```python
from build123d import *

# Parameters (mm, degrees)
ESBO_O1_R                  = 25
RESSALTO_EXTRUS_O1_DEPTH   = 22
CORTE_EXTRUS_O1_DEPTH      = 24
CORTE_EXTRUS_O1_DEPTH_BACK = 32
CORTE_EXTRUS_O2_DEPTH      = 32
PADR_OCIRCULAR1_COUNT      = 14


with BuildPart() as part:
    # Esboço1 → Ressalto-extrusão1 (new body)
    with BuildSketch(Plane.XY):
        Circle(ESBO_O1_R)
    extrude(amount=RESSALTO_EXTRUS_O1_DEPTH)

    # Esboço2 → Corte-extrusão1 (cut, two sides: drawn at the far end of the back side and taken through both)
    with BuildSketch(Plane.XY.offset(22).offset(-CORTE_EXTRUS_O1_DEPTH_BACK)):
        with BuildLine():
            Line((-2.5, -11), (2.5, -11))
            Line((2.5, -11), (2.5, -14.282856857))
            ThreePointArc((2.5, -14.282856857), (10.253048327, -10.253048327), (14.282856857, -2.5))
            Line((14.282856857, -2.5), (11, -2.5))
            Line((11, -2.5), (11, 2.5))
            Line((11, 2.5), (14.282856857, 2.5))
            ThreePointArc((14.282856857, 2.5), (10.253048327, 10.253048327), (2.5, 14.282856857))
            Line((2.5, 14.282856857), (2.5, 11))
            Line((2.5, 11), (-2.5, 11))
            Line((-2.5, 11), (-2.5, 14.282856857))
            ThreePointArc((-2.5, 14.282856857), (-10.253048327, 10.253048327), (-14.282856857, 2.5))
            Line((-14.282856857, 2.5), (-11, 2.5))
            Line((-11, 2.5), (-11, -2.5))
            Line((-11, -2.5), (-14.282856857, -2.5))
            ThreePointArc((-14.282856857, -2.5), (-10.253048327, -10.253048327), (-2.5, -14.282856857))
            Line((-2.5, -14.282856857), (-2.5, -11))
        make_face()
    extrude(amount=CORTE_EXTRUS_O1_DEPTH + CORTE_EXTRUS_O1_DEPTH_BACK, mode=Mode.SUBTRACT)

    # Esboço3 → Corte-extrusão2 (cut)
    with BuildSketch(Plane.XY.offset(22)):
        Polygon((-3.376446492, -24.770942838), (0.890947549, -26.390974492), (3.376446492, -24.770942838), (2.5, -21.5), (-2.5, -21.5), align=None)
    corte_extrus_o2 = extrude(amount=-CORTE_EXTRUS_O2_DEPTH, mode=Mode.SUBTRACT)

    # PadrãoCircular1: Corte-extrusão2 ×14 about axis
    padr_ocircular1_axis = Axis((0, 0, 0), (0, 0, 1))
    for i in range(1, PADR_OCIRCULAR1_COUNT):
        add(corte_extrus_o2.rotate(padr_ocircular1_axis, i * 360 / PADR_OCIRCULAR1_COUNT), mode=Mode.SUBTRACT)


solid = part.part
```
Source: CAD feature listing. Evaluate the final solid. Frame: model axes, mm. A direction names the side the tool comes from. Round coordinates to 2 decimals unless told otherwise and drop trailing zeros. Loops run counter-clockwise (first coordinate to the right, second up) from the corner with the lowest first, then second, coordinate; pieces in that order, holes last.
1. Ray query, L1, parallel to Y at x = 17, z = 14.75; L2, parallel to X at y = 20, z = 2.5; L3, parallel to X at y = 12, z = 2. Return the intervals inside material, ascending.
2. Section query A-A on x = -0.5. Output: boundary loops of the cut face in (y, z), and give its area (3 significant figures).
3. Section query C-C on x = 19.5. Output: boundary loops of the cut face in (y, z).
4. Contact query for flat-ended pins moving along their axis: pin 1 (1.6 mm diameter, centred on x = 12, z = 10, fed in from +Y); pin 2 (5 mm diameter, centred on y = 17.5, z = 12, fed in from +X); pin 3 (2.5 mm diameter, centred on x = -1, z = 12, fed in from +Y); pin 4 (1.5 mm diameter, centred on x = 12.5, y = 3.5, fed in from +Z). Output: stop coordinate, or through.
5. Access query for faces 1 (the cylindrical face through (5.53, -24.38, 10.85)), 2 (the flat face through (-16.27, -16.74, 11.15)), 3 (the cylindrical face through (10.165, -10.341, 10.846)), 4 (the flat face through (-19.942, 12.137, 11.154)), 5 (the flat face through (-12.67, -19.55, 11.15)). Directions: +Z, -Z, +X, -X, +Y, -Y. A direction counts if a zero-diameter tool reaches every point of the face in a straight line with its end or side. Return the directions, or none.
6. Mould query, pull axis X, two halves, no side actions, for faces 6 (the flat face through (13, -2.5, 11)), 7 (the flat face through (-21.923, -8.024, 11.154)), 8 (the cylindrical face through (15.56, -19.57, 10.85)). Classes: released by +X, released by -X, zero draft, split by the parting line, or undercut.
7. Section query B-B on y = 6.5. Output: boundary loops of the cut face in (x, z), and give its area (3 significant figures).
Answers below:
1. L1: y = -18.33 to -17.73, -13.17 to 13.17, 17.73 to 18.33
1. L2: x = -15 to -13.06, -8.02 to 8.02, 13.06 to 15
1. L3: x = -21.93 to -19.63, -17.93 to -8.14, -2.5 to 2.5, 8.14 to 17.93, 19.63 to 21.93
2. outline: (-21.5, 0) - (-11, 0) - (-11, 22) - (-21.5, 22) - close; (11, 0) - (21.5, 0) - (21.5, 22) - (11, 22) - close
2. area: 462 mm2
3. outline: (-11.94, 0) - (11.94, 0) - (11.94, 22) - (-11.94, 22) - close
4. pin 1: stops at y = 19.7
4. pin 2: stops at x = 17.26
4. pin 3: stops at y = 21.5
4. pin 4: passes through
5. face 1: +Z, -Z, +X, -Y
5. face 2: +Z, -Z, -X
5. face 3: +Z, -Z
5. face 4: +Z, -Z, +Y
5. face 5: +Z, -Z, -Y
6. face 6: undercut
6. face 7: released by -X
6. face 8: released by +X
7. outline: (-20.57, 0) - (-12.96, 0) - (-12.96, 22) - (-20.57, 22) - close; (12.96, 0) - (20.57, 0) - (20.57, 22) - (12.96, 22) - close
7. area: 335 mm2
